Here's how the part is built. I have some questions about the finished solid (model axes, mm). A direction names the side the tool comes from. Coordinates: 2 decimals unless noted, no trailing zeros. Write each loop counter-clockwise with the first axis right and the second up, starting at its lowest first coordinate (ties: lowest second). Pieces come first, ordered by that corner, then holes.
Autodesk Fusion 360 part; units mm, degrees
sketch "スケッチ1" plane through (0, 0, 0) normal (0, 0, 1) x (1, 0, 0)
  line L0 (0, 0) -> (52, 0)
  line L1 (52, 0) -> (52, 57)
  line L2 (52, 57) -> (0, 57)
  line L3 (0, 57) -> (0, 0)
  dimension "d1" = 57
extrude "押し出し1" add sketch "スケッチ1" along normal blind 30
sketch "スケッチ2" plane through (0, 0, 30) normal (0, 0, 1) x (-1, 0, 0)
  line L0 (0, -57) -> (0, 0)
  line L1 (0, 0) -> (-52, 0)
  line L2 (-52, 0) -> (-52, -57)
  line L3 (-52, -57) -> (0, -57)
  line L4 (-45, -7) -> (-45, -50)
  line L5 (-45, -50) -> (-7, -50)
  line L6 (-7, -50) -> (-7, -7)
  line L7 (-12, -7) -> (-45, -7)
  line L8 (-45, -7) -> (-50, -7)
  line L9 (-50, -12) -> (-50, -50)
  line L10 (-50, -50) -> (-45, -50)
  line L11 (-45, -50) -> (-45, -7)
  line L12 (-7, -7) -> (-45, -7)
  line L13 (-50, -7) -> (-50, -45)
  line L14 (-45, -50) -> (-12, -50)
  line L15 (-7, -45) -> (-7, -12)
  line L16 (-7, -45) -> (-12, -50)
  line L17 (-45, -50) -> (-50, -45)
  line L18 (-45, -7) -> (-50, -12)
  line L19 (-12, -7) -> (-7, -12)
  point P0 (-7, -50)
  dimension "d5" = 5
  dimension "d6" = 5
  dimension "d7" = 5
  dimension "d8" = 5
  dimension "d9" = 5
  dimension "d10" = 5
  dimension "d11" = 5
  dimension "d12" = 5
extrude "押し出し2" cut sketch "スケッチ2" against normal blind 28 contours L4 L5 L6 L7 L11 L12 L14 L15 L16 L19 | L4 L9 L11 L13 L17 L18
sketch "スケッチ3" plane through (0, 0, 30) normal (0, 0, 1) x (-1, 0, 0)
  line L0 (-50, -45) -> (-50, -12)
  line L1 (-50, -12) -> (-45, -7)
  line L2 (-45, -7) -> (-12, -7)
  line L3 (-12, -7) -> (-7, -12)
  line L4 (-7, -12) -> (-7, -45)
  line L5 (-7, -45) -> (-12, -50)
  line L6 (-12, -50) -> (-45, -50)
  line L7 (-45, -50) -> (-50, -45)
  line L8 (0, -57) -> (0, 0)
  line L9 (0, 0) -> (-52, 0)
  line L10 (-52, 0) -> (-52, -57)
  line L11 (-52, -57) -> (0, -57)
  line L12 (0, -57) -> (-26.0227, -57)
  line L13 (-26.0227, -57) -> (-26.0227, -53.5)
  line L14 (-26.0227, -53.5) -> (0, -53.5)
  line L15 (0, -53.5) -> (0, -57)
  line L16 (-26.0227, -53.5) -> (-52, -53.5)
  line L17 (-52, -53.5) -> (-52, -57)
  line L18 (-52, -57) -> (-26.0227, -57)
  line L19 (-26.0227, -57) -> (-26.0227, -53.5)
  line L20 (0, 0) -> (-26.0083, 0)
  line L21 (-26.0083, 0) -> (-26.0083, -3.5)
  line L22 (-26.0083, -3.5) -> (0, -3.5)
  line L23 (0, -3.5) -> (0, 0)
  line L24 (-26.0083, 0) -> (-52, 0)
  line L25 (-52, 0) -> (-52, -3.5)
  line L26 (-52, -3.5) -> (-26.0083, -3.5)
  line L27 (-26.0083, -3.5) -> (-26.0083, 0)
  line L28 (0, -57) -> (-5, -57)
  line L29 (-5, -57) -> (-5, -53.5)
  line L30 (-5, -53.5) -> (0, -53.5)
  line L31 (0, -53.5) -> (0, -57)
  line L32 (-52, -57) -> (-47, -57)
  line L33 (-47, -57) -> (-47, -53.5)
  line L34 (-47, -53.5) -> (-52, -53.5)
  line L35 (-52, -53.5) -> (-52, -57)
  line L36 (0, 0) -> (-5, 0)
  line L37 (-5, 0) -> (-5, -3.5)
  line L38 (-5, -3.5) -> (0, -3.5)
  line L39 (0, -3.5) -> (0, 0)
  line L40 (-52, 0) -> (-47, 0)
  line L41 (-47, 0) -> (-47, -3.5)
  line L42 (-47, -3.5) -> (-52, -3.5)
  line L43 (-52, -3.5) -> (-52, 0)
  line L44 (-26.0227, -53.5) -> (-30.042, -53.5)
  line L45 (-30.042, -53.5) -> (-30.042, -57)
  line L46 (-30.042, -57) -> (-26.0227, -57)
  line L47 (-26.0227, -57) -> (-26.0227, -53.5)
  line L48 (-26.0227, -53.5) -> (-22.0467, -53.5)
  line L49 (-22.0467, -53.5) -> (-22.0467, -57)
  line L50 (-22.0467, -57) -> (-26.0227, -57)
  line L51 (-26.0227, -57) -> (-26.0227, -53.5)
  line L52 (-26.0083, 0) -> (-30.0469, 0)
  line L53 (-30.0469, 0) -> (-30.0469, -3.5)
  line L54 (-30.0469, -3.5) -> (-26.0083, -3.5)
  line L55 (-26.0083, -3.5) -> (-26.0083, 0)
  line L56 (-26.0083, 0) -> (-22.0451, 0)
  line L57 (-22.0451, 0) -> (-22.0451, -3.5)
  line L58 (-22.0451, -3.5) -> (-26.0083, -3.5)
  line L59 (-26.0083, -3.5) -> (-26.0083, 0)
  circle A0 centre (-5, -53.5) radius 2.25
  circle A1 centre (-22.0467, -53.5) radius 2.25
  circle A2 centre (-30.042, -53.5) radius 2.25
  circle A3 centre (-47, -53.5) radius 2.25
  circle A4 centre (-5, -3.5) radius 2.25
  circle A5 centre (-22.0451, -3.5) radius 2.25
  circle A6 centre (-30.0469, -3.5) radius 2.25
  circle A7 centre (-47, -3.5) radius 2.25
  dimension "d15" = 3.5
  dimension "d16" = 3.5
  dimension "d17" = 3.5
  dimension "d18" = 4.5
  dimension "d19" = 4.5
  dimension "d20" = 4.5
  dimension "d21" = 4.5
  dimension "d22" = 4.5
  dimension "d23" = 4.5
  dimension "d24" = 4.5
  dimension "d25" = 4.5
extrude "押し出し3" cut sketch "スケッチ3" against normal blind 6 contours L14 L29 L30 A0 | L14 L30 A0 | L14 L29 A0 | L22 L38 A4 | L22 L37 L38 A4 | L14 L48 L49 A1 | L14 L49 A1 | L22 L37 A4 | L14 L48 A1 | L22 L58 A5 | L22 L57 A5 | L16 L45 A2 | L16 L44 L45 A2 | L16 L44 A2 | L22 L57 L58 A5 | L16 L33 L34 A3 | L16 L33 A3 | L16 L34 A3 | L26 L53 L54 A6 | L26 L53 A6 | L26 L54 A6 | L26 L41 A7 | L26 L41 L42 A7 | L26 L42 A7
sketch "スケッチ4" plane through (0, 0, 24) normal (0, 0, 1) x (-1, 0, 0)
  circle A0 centre (-5, -53.5) radius 2.25
  circle A1 centre (-5, -53.5) radius 1.65
  circle A2 centre (-5, -3.5) radius 1.65
  circle A3 centre (-47, -3.5) radius 1.65
  circle A4 centre (-47, -53.5) radius 1.65
  dimension "d28" = 3.3
  dimension "d29" = 3.3
  dimension "d30" = 3.3
  dimension "d31" = 3.3
extrude "押し出し4" cut sketch "スケッチ4" against normal blind 24 contours A1 | A2 | A3 | A4
sketch "スケッチ5" plane through (0, 0, 0) normal (-1, 0, 0) x (0, -1, 0)
  line L0 (-57, 0) -> (0, 0)
  line L1 (0, 0) -> (0, 30)
  line L2 (0, 30) -> (-57, 30)
  line L3 (-57, 30) -> (-57, 0)
  line L4 (-57, 0) -> (-28.5, 0)
  line L5 (-28.5, 0) -> (-28.5, 2)
  line L6 (-28.5, 2) -> (-57, 2)
  line L7 (-57, 2) -> (-57, 0)
  line L8 (-28.5, 2) -> (-14.5, 2)
  line L9 (-14.5, 2) -> (-14.5, 30)
  line L10 (-14.5, 30) -> (-28.5, 30)
  line L11 (-28.5, 30) -> (-28.5, 2)
  line L12 (-28.5, 2) -> (-42.5, 2)
  line L13 (-42.5, 2) -> (-42.5, 30)
  line L14 (-42.5, 30) -> (-28.5, 30)
  line L15 (-28.5, 30) -> (-28.5, 2)
  dimension "d34" = 28.5
  dimension "d35" = 2
  dimension "d36" = 14
  dimension "d37" = 28
  dimension "d38" = 14
  dimension "d39" = 28
extrude "押し出し5" cut sketch "スケッチ5" against normal blind 7 contours L2 L8 L9 L10 L11 L15 | L2 L6 L11 L12 L13 L14 L15
sketch "スケッチ6" plane through (0, 0, 0) normal (0, -1, 0) x (1, 0, 0)
  line L0 (0, 0) -> (52, 0)
  line L1 (52, 0) -> (52, 30)
  line L2 (52, 30) -> (0, 30)
  line L3 (0, 30) -> (0, 0)
  line L4 (0, 30) -> (15, 30)
  line L5 (15, 30) -> (15, 0)
  line L6 (15, 0) -> (0, 0)
  line L7 (0, 0) -> (0, 30)
  line L8 (52, 0) -> (37, 0)
  line L9 (37, 0) -> (37, 30)
  line L10 (37, 30) -> (52, 30)
  line L11 (52, 30) -> (52, 0)
  line L12 (0, 30) -> (52, 30)
  line L13 (52, 30) -> (52, 23)
  line L14 (52, 23) -> (0, 23)
  line L15 (0, 23) -> (0, 30)
  line L16 (0, 0) -> (52, 0)
  line L17 (52, 0) -> (52, 7)
  line L18 (52, 7) -> (0, 7)
  line L19 (0, 7) -> (0, 0)
  dimension "d42" = 15
  dimension "d43" = 30
  dimension "d44" = 15
  dimension "d45" = 30
  dimension "d46" = 7
  dimension "d47" = 7
extrude "押し出し6" cut sketch "スケッチ6" against normal blind 7 contours L5 L9 L14 L18
sketch "スケッチ7" plane through (0, 57, 0) normal (0, 1, 0) x (-1, 0, 0)
  line L0 (-52, 0) -> (0, 0)
  line L1 (0, 0) -> (0, 30)
  line L2 (0, 30) -> (-52, 30)
  line L3 (-52, 30) -> (-52, 0)
  line L4 (-52, 0) -> (-37, 0)
  line L5 (-37, 0) -> (-37, 30)
  line L6 (-37, 30) -> (-52, 30)
  line L7 (-52, 30) -> (-52, 0)
  line L8 (0, 0) -> (-15, 0)
  line L9 (-15, 0) -> (-15, 30)
  line L10 (-15, 30) -> (0, 30)
  line L11 (0, 30) -> (0, 0)
  line L12 (-52, 30) -> (0, 30)
  line L13 (0, 30) -> (0, 23)
  line L14 (0, 23) -> (-52, 23)
  line L15 (-52, 23) -> (-52, 30)
  line L16 (-52, 0) -> (0, 0)
  line L17 (0, 0) -> (0, 7)
  line L18 (0, 7) -> (-52, 7)
  line L19 (-52, 7) -> (-52, 0)
  dimension "d50" = 15
  dimension "d51" = 30
  dimension "d52" = 15
  dimension "d53" = 30
  dimension "d54" = 7
  dimension "d55" = 7
extrude "押し出し7" cut sketch "スケッチ7" against normal blind 7 contours L5 L9 L14 L18
equation "d6 = d5"
equation "d8 = d7"
equation "d10 = d9"
equation "d12 = d11"
1) On a 3-axis mill with a long thin cutter (end or side, diameter ignored), from which of +Z, -Z, +X, -X, +Y, -Y can I reach the whole of each face in a straight line? I mean faces 1 (the face through (26, 52, 30)), 2 (the face through (37, 54, 15)), 3 (the face through (49.248, 3.401, 27.042)). Say none if no direction works.
Values follow:
face 1: +Z, +X, -X, +Y, -Y
face 2: +Y, -Y
face 3: +Z
2) Imagine slicing it at A-A on x = 5. Please give me the cut outline in (y, z).
Values follow:
outline: (0, 0) - (1.85, 0) - (1.85, 24) - (1.25, 24) - (1.25, 30) - (0, 30) - close; (5.15, 0) - (51.85, 0) - (51.85, 24) - (51.25, 24) - (51.25, 30) - (42.5, 30) - (42.5, 2) - (14.5, 2) - (14.5, 30) - (5.75, 30) - (5.75, 24) - (5.15, 24) - close; (55.15, 0) - (57, 0) - (57, 30) - (55.75, 30) - (55.75, 24) - (55.15, 24) - close
3) Imagine slicing it at C-C on y = 3.5. Count the separate pieces of the cut face and the enclosed holes in it, then the cut area to 3 significant figures.
Values follow:
separate pieces: 3
enclosed holes: 1
area: 942 mm2
4) Imagine slicing it at B-B on z = 8.5. Please give me the cut outline in (x, y), then the cut area to 3 significant figures.
Values follow:
outline: (0, 0) - (15, 0) - (15, 7) - (12, 7) - (7, 12) - (7, 14.5) - (0, 14.5) - close; (0, 42.5) - (7, 42.5) - (7, 45) - (12, 50) - (15, 50) - (15, 57) - (0, 57) - close; (37, 0) - (52, 0) - (52, 57) - (37, 57) - (37, 50) - (45, 50) - (50, 45) - (50, 12) - (45, 7) - (37, 7) - close; hole circle Ø3.3 at (5, 3.5); hole circle Ø3.3 at (5, 53.5); hole circle Ø3.3 at (47, 3.5); hole circle Ø3.3 at (47, 53.5)
area: 627 mm2
5) Imagine slicing it at D-D on z = 4.25. Please give me the cut outline in (x, y).
Values follow:
outline: (0, 0) - (52, 0) - (52, 57) - (0, 57) - (0, 42.5) - (7, 42.5) - (7, 45) - (12, 50) - (45, 50) - (50, 45) - (50, 12) - (45, 7) - (12, 7) - (7, 12) - (7, 14.5) - (0, 14.5) - close; hole circle Ø3.3 at (5, 3.5); hole circle Ø3.3 at (5, 53.5); hole circle Ø3.3 at (47, 3.5); hole circle Ø3.3 at (47, 53.5)
6) Will these pins go through, and if not, where does the flat tip stop? pin 1 (3.5 mm diameter, centred on x = 22, y = 53.5, fed in from +Z); pin 2 (4 mm diameter, centred on x = 45.5, y = 29.5, fed in from +Z).
Values follow:
pin 1: stops at z = 24
pin 2: stops at z = 2
7) We'd pull the mould along X, two halves only. Please class faces 4 (the face through (15, 3, 15)), 5 (the face through (52, 28, 15)), 6 (the face through (0, 29, 1)): pulls with the +X half, pulls with the -X half, needs draft (parallel to the pull), parting line crosses it, or undercut.
Values follow:
face 4: undercut
face 5: pulls with the +X half
face 6: pulls with the -X half
8) I need wall thicknesses on probe 1 along X at (y, z) = (53.5, 26.6); probe 2 along Y at (x, z) = (5, 7.5); probe 3 along X at (y, z) = (53.5, 9). Which ranges of each line are inside material? Lowest first, please.
Values follow:
probe 1: x = 0 to 2.75, 7.25 to 19.8, 24.3 to 27.79, 32.29 to 44.75, 49.25 to 52
probe 2: y = 0 to 1.85, 5.15 to 14.5, 42.5 to 51.85, 55.15 to 57
probe 3: x = 0 to 3.35, 6.65 to 15, 37 to 45.35, 48.65 to 52
